For this review, take the finished solid that the model builds, in its own axes (mm). Face numbers are marked on the shaded views. A direction names the side the tool comes from. Give positions to 0.01 mm unless a question says otherwise; leave off trailing zeros. Loops run counter-clockwise (first coordinate to the right, second up) from the corner with the lowest first, then second, coordinate; pieces in that order, holes last. Notation, with made-up numbers: (86, -26.75) - (113, -26.75) arc R14 cw to (113, -9.75) - close; hole circle Ø3 at (-4.75, 67.25). An arc over 180 degrees is marked (long way). Answer in a Markdown table with one row per item.
```python
from build123d import *

# Parameters (mm, degrees)
BOSS_EXTRUDE1_DEPTH = 6.35
SKETCH3_R           = 3.175
BOSS_EXTRUDE2_DEPTH = 12.7
FILLET1_R           = 3.175
SKETCH4_R           = 5.136753641
BOSS_EXTRUDE3_DEPTH = 9.525
BOSS_EXTRUDE3_TAPER = 3


with BuildPart() as part:
    # Sketch1 → Boss-Extrude1 (new body)
    with BuildSketch(Plane(origin=(0, 0, 0), x_dir=(1, 0, 0), z_dir=(0, 1, 0))):
        Polygon((5.55625, 3.207902433), (0, 6.415804866), (-5.55625, 3.207902433), (-5.55625, -3.207902433), (0, -6.415804866), (5.55625, -3.207902433), align=None)
    extrude(amount=BOSS_EXTRUDE1_DEPTH)

    # Sketch3 → Boss-Extrude2 (add)
    with BuildSketch(Plane(origin=(0, 6.35, 0), x_dir=(1, 0, 0), z_dir=(0, 1, 0))):
        with Locations(Location((0, 0, 0), (0, 0, 270))):
            Circle(SKETCH3_R)
    extrude(amount=BOSS_EXTRUDE2_DEPTH)

    # Fillet1
    fillet1_edges = [part.edges().sort_by_distance(p)[0] for p in [
        (0, 19.05, -3.175),
    ]]
    fillet(fillet1_edges, radius=FILLET1_R)

    # Sketch4 → Boss-Extrude3 (add)
    with BuildSketch(Plane.XZ):
        Circle(SKETCH4_R)
    extrude(amount=BOSS_EXTRUDE3_DEPTH, taper=BOSS_EXTRUDE3_TAPER)


solid = part.part
```
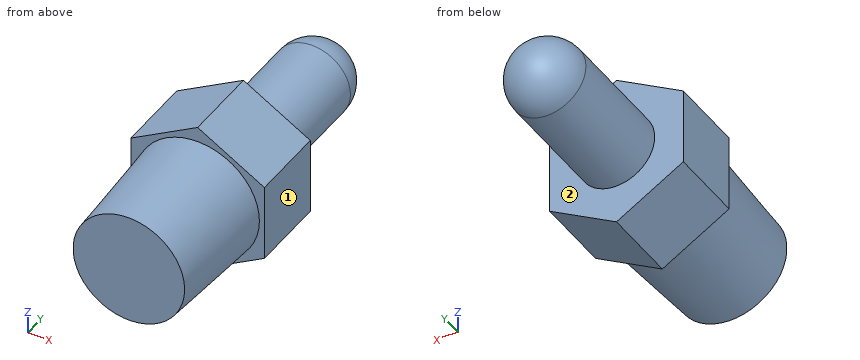
1. For the marked faces 1 and 2, list the 3-axis set-ups (+Z, -Z, +X, -X, +Y, -Y) from which the entire face can be reached by the end or side of a thin tool; tool diameter is ignored.
Values:
| item | result |
|---|---|
| face 1 | +Z, -Z, +X, +Y, -Y |
| face 2 | +Y |
2. Clearance check with flat-ended pins moving along their axes: pin 1 (2 mm diameter, centred on x = -3.5, z = 4.5, fed in from +Y); pin 2 (1.5 mm diameter, centred on x = -0.5, z = -3.5, fed in from +Y); pin 3 (3.5 mm diameter, centred on x = -2.5, z = 0, fed in from +Y). State where each tip first meets the part, or that it passes through.
Values:
| item | result |
|---|---|
| pin 1 | stops at y = 6.35 |
| pin 2 | stops at y = 17.4 |
| pin 3 | stops at y = 18.96 |
3. Wall thickness on line 1 (Y direction, x = -4.25, z = 1) (3 decimals); line 2 (Y direction, x = -1.75, z = -5); line 3 (Z direction, x = -1.5, y = 6): over which ranges is each line inside the solid? List them lowest first. Write a range as [from, to].
Values:
| item | result |
|---|---|
| line 1 | y = [-9.525, 6.35] |
| line 2 | y = [0, 6.35] |
| line 3 | z = [-5.55, 5.55] |
4. We need section A-A, the plane y = 17. Give the boundary of the cut face in (x, z).
Values:
| item | result |
|---|---|
| outline | circle Ø5.94 at (0, 0) |
